Geometry check sheet. Reference: the model listing, model coordinates, mm. Face numbers are marked on the shaded views. A direction names the side the tool comes from. Round coordinates to 2 decimals unless told otherwise and drop trailing zeros. Loops run counter-clockwise (first coordinate to the right, second up) from the corner with the lowest first, then second, coordinate; pieces in that order, holes last. Notation, with made-up numbers: (-21.5, -4.75) - (34.5, -4.75) arc R20 ccw to (34.5, 24.25) - close; hole circle Ø6 at (15.25, 9). An arc over 180 degrees is marked (long way). Write item = value, one per line.
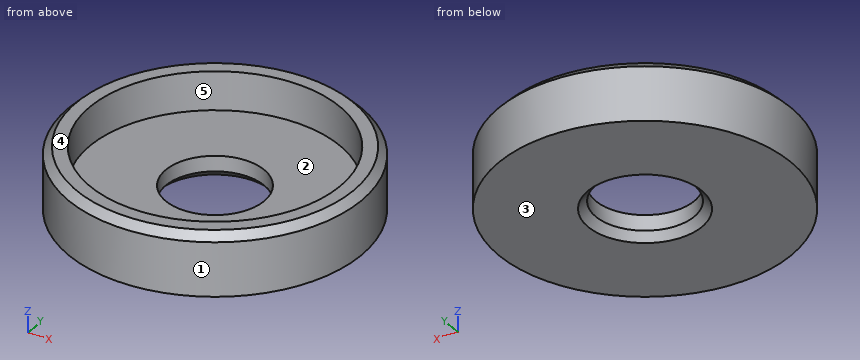
Autodesk Fusion 360 part; units mm, degrees
sketch "Sketch1" plane through (0, 0, 0) normal (0, 0, 1) x (1, 0, 0)
  circle A0 centre (0, 0) radius 16.25
  circle A1 centre (0, 0) radius 19
  circle A2 centre (0, 0) radius 6.4
  dimension "d1" = 32.5
  dimension "d2" = 38
  dimension "d3" = 12.8
extrude "Extrude1" add sketch "Sketch1" along normal blind 8 contours A1
extrude "Extrude2" add sketch "Sketch1" along normal blind 3 contours A0
chamfer "Chamfer1" distance 1 angle 45 1 edges at (-17.7142, -6.8707, 8)
chamfer "Chamfer2" distance 1 angle 45 1 edges at (-5.9669, 2.3143, 0)
(1) Scan lines: L1, parallel to Y at x = 0, z = 5.85; L2, parallel to X at y = 2.5, z = 4; L3, parallel to Y at x = -5.5, z = 5.75. Record each from-to range of solid material in increasing order. Write a range as [from, to].
Answers follow:
L1 = [-19, -16.25], [16.25, 19]
L2 = [-18.83, -16.06], [16.06, 18.83]
L3 = [-18.19, -15.29], [15.29, 18.19]
(2) Section check C-C (z = 5.25). Enter the section's corners in (x, y), then the cut area to 3 significant figures.
Answers follow:
outline = circle Ø38 at (0, 0); hole circle Ø32.5 at (0, 0)
area = 305 mm²
(3) Set-up check for the marked faces 4 and 5: record each of +Z, -Z, +X, -X, +Y, -Y from which the full face is reachable in a straight line by a thin tool's end or side.
Answers follow:
face_4 = +Z, +X, -X, +Y, -Y
face_5 = +Z
(4) Gauge pin test, flat ends, axial feed: pin 1 (10 mm diameter, centred on x = 15, y = 9.5, fed in from -Z); pin 2 (2 mm diameter, centred on y = -10.5, z = 4, fed in from +X); pin 3 (4 mm diameter, centred on x = 6, z = 6.5, fed in from -Y); pin 4 (4 mm diameter, centred on x = 2.5, z = 4, fed in from -Y). Record the tip position at first contact, or that the pin passes through.
Answers follow:
pin_1 = 0
pin_2 = 16.45
pin_3 = -18.57
pin_4 = -18.99
(5) Section check A-A (y = 0). Enter the section's corners in (x, z), then the cut area to 3 significant figures.
Answers follow:
outline = (-19, 0) - (-7.4, 0) - (-6.4, 1) - (-6.4, 3) - (-16.25, 3) - (-16.25, 8) - (-18, 8) - (-19, 7) - close; (6.4, 1) - (7.4, 0) - (19, 0) - (19, 7) - (18, 8) - (16.25, 8) - (16.25, 3) - (6.4, 3) - close
area = 101 mm²
(6) Mould release check, pull along Y, two halves, no side actions. Record for the marked faces 1, 2 and 3: pulls with the +Y half, pulls with the -Y half, needs draft (parallel to the pull), parting line crosses it, or undercut.
Answers follow:
face_1 = parting line crosses it
face_2 = undercut
face_3 = needs draft
